Check sheet for the drawn part. Datum: minimum x, y, z corner. Units: mm. A direction names the side the tool comes from. Round coordinates to 2 decimals unless told otherwise and drop trailing zeros. Loops run counter-clockwise (first coordinate to the right, second up) from the corner with the lowest first, then second, coordinate; pieces in that order, holes last.
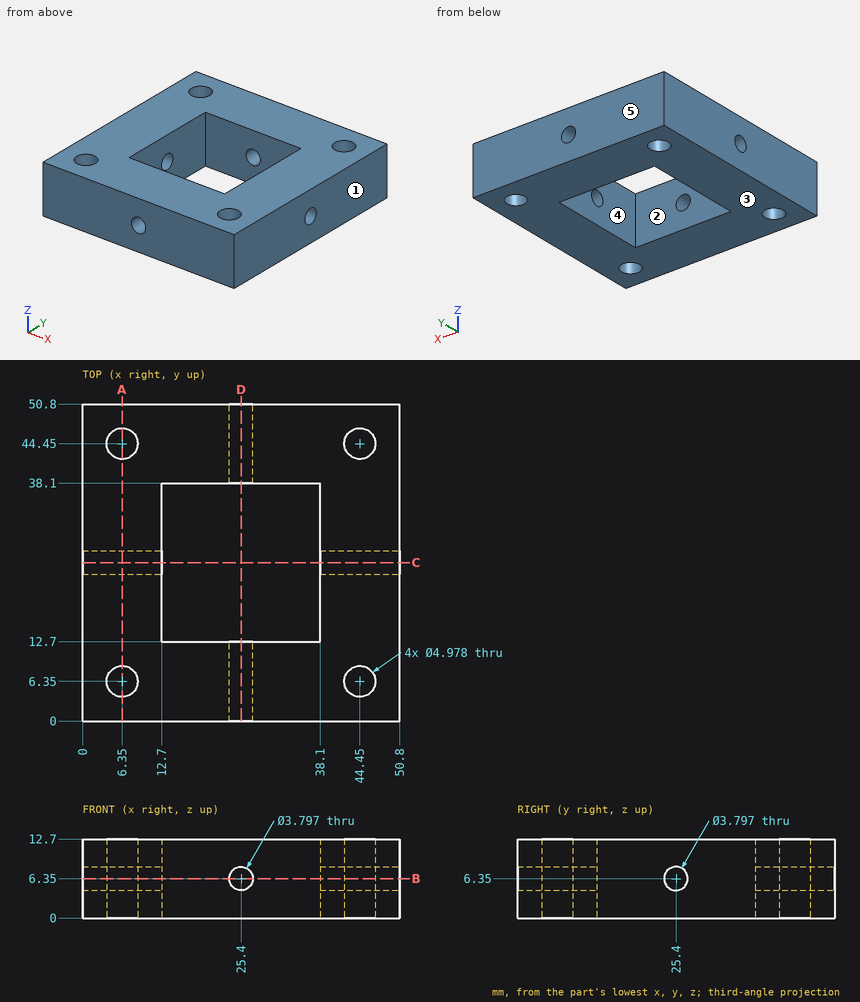
1) Sectioned sample at A-A, the plane x = 6.35. Record the cut outline in (y, z).
Report:
outline: (0, 0) - (3.86, 0) - (3.86, 12.7) - (0, 12.7) - close; (8.84, 0) - (41.96, 0) - (41.96, 12.7) - (8.84, 12.7) - close; (46.94, 0) - (50.8, 0) - (50.8, 12.7) - (46.94, 12.7) - close; hole circle Ø3.8 at (25.4, 6.35)
2) Mould release check, pull along Y, two halves, no side actions. Record for the marked faces 3, 4 and 5: +Y half, -Y half, draft (parallel to the pull), parting line (faces both ways), or undercut.
Report:
face 3: draft
face 4: undercut
face 5: +Y half
3) Sectioned sample at C-C, the plane y = 25.4. Record the cut outline in (x, z), then the cut area to 3 significant figures.
Report:
outline: (0, 0) - (12.7, 0) - (12.7, 4.45) - (0, 4.45) - close; (0, 8.25) - (12.7, 8.25) - (12.7, 12.7) - (0, 12.7) - close; (38.1, 0) - (50.8, 0) - (50.8, 4.45) - (38.1, 4.45) - close; (38.1, 8.25) - (50.8, 8.25) - (50.8, 12.7) - (38.1, 12.7) - close
area: 226 mm2
4) Gauge pin test, flat end, axial feed: pin 1 (3 mm diameter, centred on x = 25.4, z = 6.35, fed in from +Y). Record the tip position at first contact, or that the pin passes through.
Report:
pin 1: passes through
5) Access from +Z, -Z, +X, -X, +Y, -Y to the whole of each face (thin tool, end or side, straight path). Record for the marked faces 1 and 2.
Report:
face 1: +Z, -Z, +X, +Y, -Y
face 2: +Z, -Z
6) Sectioned sample at B-B, the plane z = 6.35. Record the cut outline in (x, y).
Report:
outline: (0, 0) - (23.5, 0) - (23.5, 12.7) - (12.7, 12.7) - (12.7, 23.5) - (0, 23.5) - close; (0, 27.3) - (12.7, 27.3) - (12.7, 38.1) - (23.5, 38.1) - (23.5, 50.8) - (0, 50.8) - close; (27.3, 0) - (50.8, 0) - (50.8, 23.5) - (38.1, 23.5) - (38.1, 12.7) - (27.3, 12.7) - close; (27.3, 38.1) - (38.1, 38.1) - (38.1, 27.3) - (50.8, 27.3) - (50.8, 50.8) - (27.3, 50.8) - close; hole circle Ø4.98 at (6.35, 6.35); hole circle Ø4.98 at (6.35, 44.45); hole circle Ø4.98 at (44.45, 6.35); hole circle Ø4.98 at (44.45, 44.45)
7) Scan lines: line 1 along Y through (x, z) = (6.35, 10.25); line 2 along Y through (x, z) = (15, 8); line 3 along Y through (x, z) = (6.35, 6.5). Record each from-to range of solid material in increasing order.
Report:
line 1: y = 0 to 3.86, 8.84 to 41.96, 46.94 to 50.8
line 2: y = 0 to 12.7, 38.1 to 50.8
line 3: y = 0 to 3.86, 8.84 to 23.51, 27.29 to 41.96, 46.94 to 50.8
